Source: CAD feature listing. Evaluate the final solid. Frame: model axes, mm. Give positions to 0.01 mm unless a question says otherwise; leave off trailing zeros. Order: outer loops, then holes, each group sorted by start corner. A loop starts at its lowest first (then second) coordinate and runs counter-clockwise, first axis right, second up.
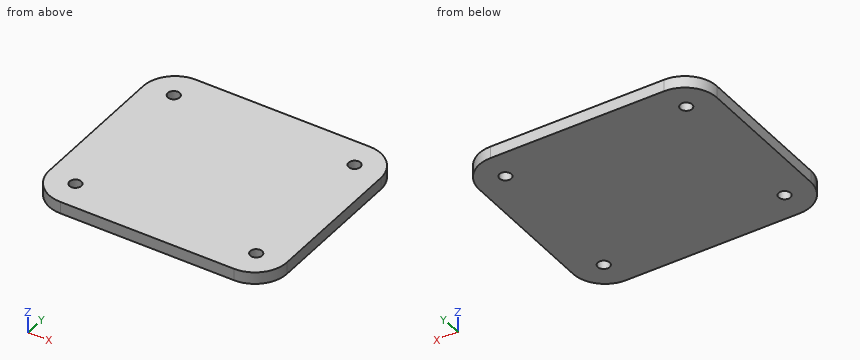
from build123d import *

# Parameters (mm, degrees)
Y_KSEKLIK_EKSTR_ZYON1_DEPTH = 5
IZIM2_R                     = 2.5
KES_EKSTR_ZYON1_DEPTH       = 10
RADYUS1_R                   = 13.5


with BuildPart() as part:
    # Çizim1 → Yükseklik-Ekstrüzyon1 (new body)
    with BuildSketch(Plane.XY):
        Polygon((21, 43.6), (50, 43.6), (50, -43.6), (-50, -43.6), (-50, 43.6), (-21, 43.6), align=None)
    extrude(amount=Y_KSEKLIK_EKSTR_ZYON1_DEPTH)

    # Çizim2 → Kes-Ekstrüzyon1 (cut)
    with BuildSketch(Plane.XY.offset(5)):
        with Locations((38, -31.6)):
            Circle(IZIM2_R)
        with Locations((38, 31.6)):
            Circle(IZIM2_R)
        with Locations((-38, 31.6)):
            Circle(IZIM2_R)
        with Locations((-38, -31.6)):
            Circle(IZIM2_R)
    extrude(amount=-KES_EKSTR_ZYON1_DEPTH, mode=Mode.SUBTRACT)

    # Radyus1
    radyus1_edges = [part.edges().sort_by_distance(p)[0] for p in [
        (50, -43.6, 2.5),
        (-50, -43.6, 2.5),
        (-50, 43.6, 2.5),
        (50, 43.6, 2.5),
    ]]
    fillet(radyus1_edges, radius=RADYUS1_R)


solid = part.part
1) Section query A-A on z = 3.6. Output: boundary loops of the cut face in (x, y), and give its area (4 significant figures).
Checks:
outline: (-50, -30.1) arc R13.5 ccw to (-36.5, -43.6) - (36.5, -43.6) arc R13.5 ccw to (50, -30.1) - (50, 30.1) arc R13.5 ccw to (36.5, 43.6) - (-36.5, 43.6) arc R13.5 ccw to (-50, 30.1) - close; hole circle Ø5 at (-38, -31.6); hole circle Ø5 at (-38, 31.6); hole circle Ø5 at (38, -31.6); hole circle Ø5 at (38, 31.6)
area: 8,485 mm2
2) Section query C-C on x = -38. Output: boundary loops of the cut face in (y, z), and give its area (3 significant figures).
Checks:
outline: (-43.52, 0) - (-34.1, 0) - (-34.1, 5) - (-43.52, 5) - close; (-29.1, 0) - (29.1, 0) - (29.1, 5) - (-29.1, 5) - close; (34.1, 0) - (43.52, 0) - (43.52, 5) - (34.1, 5) - close
area: 385 mm2
3) Section query B-B on y = 31.6. Output: boundary loops of the cut face in (x, z), and give its area (3 significant figures).
Checks:
outline: (-49.92, 0) - (-40.5, 0) - (-40.5, 5) - (-49.92, 5) - close; (-35.5, 0) - (35.5, 0) - (35.5, 5) - (-35.5, 5) - close; (40.5, 0) - (49.92, 0) - (49.92, 5) - (40.5, 5) - close
area: 449 mm2
4) First-contact query: pin 1 Ø5 at (x, y) = (-19, -27) entering from -Z. Flat tip, straight axial feed; report the tip coordinate or a pass-through.
Checks:
pin 1: stops at z = 0
5) Ray query, L1, parallel to Y at x = -38, z = 3.65; L2, parallel to Y at x = -37, z = 4.35; L3, parallel to Y at x = 42.5, z = 3.7. Return the intervals inside material, ascending.
Checks:
L1: y = -43.52 to -34.1, -29.1 to 29.1, 34.1 to 43.52
L2: y = -43.59 to -33.89, -29.31 to 29.31, 33.89 to 43.59
L3: y = -42.19 to 42.19
